```python
from build123d import *

# Parameters (mm, degrees)
SKETCH2_R           = 3.175
BOSS_EXTRUDE1_DEPTH = 2.54
SKETCH3_R           = 3.175
BOSS_EXTRUDE2_DEPTH = 2.54
SKETCH4_W           = 3.81
SKETCH4_H           = 25.4
BOSS_EXTRUDE3_DEPTH = 48.6
BOSS_EXTRUDE4_DEPTH = 50.8
LPATTERN1_COUNT     = 2
LPATTERN1_PITCH     = 19.05
SKETCH6_W           = 48.6
SKETCH6_H           = 71.12
CUT_EXTRUDE1_DEPTH  = 1.27
BOSS_EXTRUDE5_REACH = 106.623
FILLET1_R           = 8.89
FILLET2_R           = 1.27
CHAMFER1_SIZE       = 2.286
CHAMFER1_SIZE_2     = 1.319822715


# Some blends are built 0.0001 mm under size
with BuildPart() as part:
    # Sketch2 → Boss-Extrude1 (new body)
    with BuildSketch(Plane.XY):
        Polygon((0, -12.7), (63.5, -12.7), (63.5, 12.7), (0, 12.7), (-10.998522628, 12.7), (-10.998522628, 6.35), align=None)
        Circle(SKETCH2_R, mode=Mode.SUBTRACT)
        with Locations((17.78, 0)):
            Circle(SKETCH2_R, mode=Mode.SUBTRACT)
        with Locations((35.56, 0)):
            Circle(SKETCH2_R, mode=Mode.SUBTRACT)
        with Locations((53.34, 0)):
            Circle(SKETCH2_R, mode=Mode.SUBTRACT)
    extrude(amount=BOSS_EXTRUDE1_DEPTH)



with BuildPart() as body_2:
    # Sketch3 → Boss-Extrude2 (new body)
    with BuildSketch(Plane(origin=(0, 0, -48.6), x_dir=(-1, 0, 0), z_dir=(0, 0, -1))):
        Polygon((10.998522628, 12.7), (-63.5, 12.7), (-63.5, -12.7), (0, -12.7), (10.998522628, 6.35), align=None)
        with Locations(Location((0, 0, 0), (0, 0, 180))):
            Circle(SKETCH3_R, mode=Mode.SUBTRACT)
        with Locations(Location((-53.34, 0, 0), (0, 0, 180))):
            Circle(SKETCH3_R, mode=Mode.SUBTRACT)
        with Locations(Location((-35.56, 0, 0), (0, 0, 180))):
            Circle(SKETCH3_R, mode=Mode.SUBTRACT)
        with Locations(Location((-17.78, 0, 0), (0, 0, 180))):
            Circle(SKETCH3_R, mode=Mode.SUBTRACT)
    extrude(amount=BOSS_EXTRUDE2_DEPTH)


with BuildPart() as part_1:
    add(part.part)

    add(body_2.part)  # Boss-Extrude3 merges body 2
    # Sketch4 → Boss-Extrude3 (add)
    with BuildSketch(Plane(origin=(0, 0, 0), x_dir=(-1, 0, 0), z_dir=(0, 0, -1))):
        with Locations((-61.595, 0)):
            Rectangle(SKETCH4_W, SKETCH4_H)
    boss_extrude3 = extrude(amount=BOSS_EXTRUDE3_DEPTH)

    # Sketch5 → Boss-Extrude4 (add)
    with BuildSketch(Plane.XZ.offset(12.7)):
        Polygon((59.69, -48.6), (59.69, 0), (59.69, 2.54), (63.5, 2.54), (63.5, -51.14), (59.69, -51.14), align=None)
    extrude(amount=BOSS_EXTRUDE4_DEPTH)

    # LPattern1: Boss-Extrude3 ×2
    with Locations(*[(-i * LPATTERN1_PITCH, 0, 0) for i in range(1, LPATTERN1_COUNT)]):
        add(boss_extrude3)

    # Sketch6 → Cut-Extrude1 (cut)
    with BuildSketch(Plane(origin=(63.5, 0, 0), x_dir=(0, 0, -1), z_dir=(1, 0, 0))):
        with Locations((24.3, -25.4)):
            Rectangle(SKETCH6_W, SKETCH6_H)
    extrude(amount=-CUT_EXTRUDE1_DEPTH, mode=Mode.SUBTRACT)

    # Boss-Extrude5: up to this face of the body (flat: up to its plane)
    boss_extrude5_end = Plane(part_1.part.faces().sort_by_distance((31.808357107, -3.617906471, -51.14))[0])
    # Sketch7 → Boss-Extrude5 (add, up to the picked face)
    with BuildSketch(Plane.XY.offset(2.54), mode=Mode.PRIVATE) as boss_extrude5_sk1:
        Polygon((40.64, -12.7), (59.69, -31.75), (59.69, -12.7), align=None)
    boss_extrude5_tool1 = split(extrude(boss_extrude5_sk1.sketch, amount=-BOSS_EXTRUDE5_REACH, mode=Mode.PRIVATE), bisect_by=boss_extrude5_end, keep=Keep.BOTH, mode=Mode.PRIVATE)
    add(boss_extrude5_tool1.solids().sort_by(Axis((53.34, -19.05, 2.54), (0, 0, -1)))[0])

    # Fillet1
    fillet1_edges = [part_1.edges().sort_by_distance(p)[0] for p in [
        (40.64, -12.7, -24.3),
    ]]
    fillet(fillet1_edges, radius=FILLET1_R)

    # Fillet2
    fillet2_edges = [part_1.edges().sort_by_distance(p)[0] for p in [
        (20.32, -12.7, -51.14),
        (50.165, -22.225, 2.54),
        (50.165, -22.225, -51.14),
        (59.69, -31.75, -24.3),
        (20.32, -12.7, 0),
        (20.32, -12.7, 2.54),
        (63.5, -25.4, 2.54),
        (63.5, -25.4, -51.14),
        (59.69, -47.625, -51.14),
        (59.69, -47.625, 2.54),
        (59.69, -63.5, -24.3),
        (63.5, -63.5, -24.3),
        (20.32, -12.7, -48.6),
    ]]
    fillet(fillet2_edges, radius=FILLET2_R - 0.0001)  # a hair under: the kernel refuses the full size

    # Chamfer1
    # the kernel refuses this chamfer: 2.286, 1.319822715 mm, written as the material it adds along each edge
    with BuildSketch(Plane(origin=(62.23, -60.96, 0), x_dir=(-0.01932676561270189, 0.9998132206222078, 0), z_dir=(0, 0, -1))) as chamfer1_piece_1_section:
        Polygon((CHAMFER1_SIZE * 0.999813220622, CHAMFER1_SIZE * 0.0193267656127), (-CHAMFER1_SIZE_2 * 0.0193267656181, CHAMFER1_SIZE_2 * 0.999813220901), (0, 0), align=None)
    chamfer1_piece_1 = extrude(amount=48.6, mode=Mode.PRIVATE)
    chamfer1_piece_1 = split(chamfer1_piece_1, bisect_by=Plane(origin=(63.5, -60.18781376, -24.3), z_dir=(-1, 0, 0)), keep=Keep.TOP, mode=Mode.PRIVATE)
    add(chamfer1_piece_1)


solid = part_1.part
```
For this review, take the finished solid that the model builds, in its own axes (mm). A direction names the side the tool comes from. Give positions to 0.01 mm unless a question says otherwise; leave off trailing zeros. Order: outer loops, then holes, each group sorted by start corner. A loop starts at its lowest first (then second) coordinate and runs counter-clockwise, first axis right, second up.
1) For faces 4 (the face through (59.69, -47, -24)), 5 (the face through (52, -12.7, -24)), 6 (the face through (41.336, -12.465, -24.64)), 7 (the face through (62.856, -59.758, -23.96)), 8 (the face through (31, -3, -51.14)), list the 3-axis set-ups (+Z, -Z, +X, -X, +Y, -Y) from which the entire face can be reached by the end or side of a thin tool; tool diameter is ignored.
2) Take a section at C-C (z = -4). Give the boundary of the cut face in (x, y).
3) The part is to be moulded in two halves that separate along X. For faces 1 (the face through (62.23, -24, -24)), 2 (the face through (32.39, -0.14, -49.85)), 3 (the face through (-10.999, 9, -50)), say which applies: released by +X, released by -X, zero draft, split by the parting line, or undercut.
4) Insertion check: pin 1 (8.5 mm diameter, centred on x = 53.34, y = 0, fed in from +Z); pin 2 (4 mm diameter, centred on y = -1, z = -35.5, fed in from +X); pin 3 (12 mm diameter, centred on y = -48, z = -31, fed in from -X); pin 4 (6.5 mm diameter, centred on y = 6, z = -32, fed in from -X). Each pin has a flat end and moves straight along its axis. Give the tip position at first contact, or say it passes through.
5) Take a section at A-A (x = 17.78). State how many separate pieces and enclosed holes the cut face has, then the cut area to 3 significant figures.
6) Take a section at B-B (y = -55). Give the boundary of the cut face in (x, z).
7) Wall thickness on line 1 (Y direction, x = 35.56, z = 1.05) (3 decimals); line 2 (Z direction, x = 50, y = -7.5); line 3 (X direction, y = -9, z = -23.5): over which ranges is each line inside the solid? List them lowest first.
Derived:
1. face 4: +Z, -Z, -X, -Y
1. face 5: +Y
1. face 6: -X, -Y
1. face 7: +X
1. face 8: -Z, +X, -X, +Y, -Y
2. outline: (40.64, -9.02) arc R8.89 ccw to (43.24, -15.3) - (59.32, -31.38) arc R1.27 cw to (59.69, -32.28) - (59.69, -62.23) arc R1.27 ccw to (60.96, -63.5) - (62.23, -63.5) arc R1.27 ccw to (63.5, -62.23) - (63.5, -60.87) - (62.23, -58.67) - (62.23, 10.16) - (63.5, 10.16) - (63.5, 12.7) - (59.69, 12.7) - (59.69, -12.7) - (44.45, -12.7) - (44.45, 12.7) - (40.64, 12.7) - close
3. face 1: released by +X
3. face 2: undercut
3. face 3: released by -X
4. pin 1: stops at z = 2.54
4. pin 2: stops at x = 62.23
4. pin 3: stops at x = 59.69
4. pin 4: stops at x = 40.64
5. separate pieces: 4
5. enclosed holes: 0
5. area: 95.4 mm2
6. outline: (59.69, -49.87) arc R1.27 ccw to (60.96, -51.14) - (62.23, -51.14) arc R1.27 ccw to (63.5, -49.87) - (63.5, -48.6) - (62.23, -48.6) - (62.23, 0) - (63.5, 0) - (63.5, 1.27) arc R1.27 ccw to (62.23, 2.54) - (60.96, 2.54) arc R1.27 ccw to (59.69, 1.27) - close
7. line 1: y = -12.681 to -3.175, 3.175 to 12.7
7. line 2: z = -51.14 to -48.6, 0 to 2.54
7. line 3: x = 40.64 to 44.45, 59.69 to 62.23
